Here's how the part is built. I have some questions about the finished solid (model axes, mm). A direction names the side the tool comes from. Round coordinates to 2 decimals unless told otherwise and drop trailing zeros. Loops run counter-clockwise (first coordinate to the right, second up) from the corner with the lowest first, then second, coordinate; pieces in that order, holes last. Notation, with made-up numbers: M 31.25,25.5 L 36.25,25.5 A13 cw 36.25,39.5 Z; hole C 86.5,30.25 d3. An arc over 180 degrees is marked long. Use a Markdown table: item, result.
Autodesk Inventor part; units mm, degrees
ref_plane "YZ Plane" through (0, 0, 0) normal (1, 0, 0) x (0, 1, 0)
ref_plane "XZ Plane" through (0, 0, 0) normal (0, 1, 0) x (-1, 0, 0)
ref_plane "XY Plane" through (0, 0, 0) normal (0, 0, 1) x (1, 0, 0)
sketch "Sketch1" plane through (0, 0, 0) normal (0, 0, 1) x (1, 0, 0)
  line L0 (-33, 0) -> (33, 0)
  line L1 (33, 0) -> (33, -58)
  line L2 (33, -58) -> (-33, -58)
  line L3 (-33, -58) -> (-33, 0)
  point P0 (0, 0)
  dimension "d0" = 58
  dimension "d1" = 66
  dimension "d2" = 33
  dimension "d3" = 0
extrude "clamp_base" add sketch "Sketch1" against normal blind 190
sketch "Sketch2" plane through (0, 0, 0) normal (0, 0, 1) x (1, 0, 0)
  line L0 (-25, -58) -> (25, -58)
  line L1 (25, -58) -> (25, -8)
  line L2 (25, -8) -> (-25, -8)
  line L3 (-25, -8) -> (-25, -58)
  line L4 (-33, -58) -> (33, -58)
  point P0 (0, 0)
  dimension "d6" = 50
  dimension "d7" = 50
  dimension "d8" = 25
extrude "clamp_extrusion" cut sketch "Sketch2" against normal through all
sketch "Sketch4" plane through (-33, 0, 0) normal (0, 1, 0) x (1, 0, 0)
  line L0 (-70, 190) -> (101, 190)
  line L1 (101, 190) -> (101, 0)
  line L2 (101, 0) -> (-70, 0)
  line L3 (-70, 0) -> (-70, 190)
  line L4 (66, 0) -> (0, 0)
  line L5 (0, 190) -> (66, 190)
  line L6 (0, 0) -> (0, 190)
  line L7 (66, 0) -> (66, 190)
  point P0 (33, 0)
  dimension "d35" = 0
  dimension "d36" = 0
  dimension "d37" = 70
  dimension "d38" = 35
extrude "platform" add sketch "Sketch4" along normal blind 15
sketch "Sketch8" plane through (33, -58, 0) normal (1, 0, 0) x (0, 0, -1)
  line L0 (0, 0) -> (0, 58)
  line L1 (190, 58) -> (190, 0)
  point P0 (45, 24.0271)
  point P1 (145, 24.0271)
  dimension "d51" = 45
  dimension "d60" = 100
  dimension "d61" = 190
hole "clampHole" at (33, -33.9729, -45) at (33, -33.9729, -145) direction (-1, 0, 0) diameter 10 end through all
sketch "tabWeld" plane through (-33, 15, 0) normal (0, 1, 0) x (1, 0, 0)
  line L0 (6.168, 65.1137) -> (67.4515, 116.5367)
  line L1 (-26.6142, 104.1819) -> (34.6693, 155.6049)
  line L2 (-70, 0) -> (101, 0)
  line L3 (-70, 190) -> (-70, 0)
  line L4 (6.168, 65.1137) -> (-26.6142, 104.1819)
  line L5 (-10.2231, 84.6478) -> (51.0604, 136.0708)
  line L6 (101, 0) -> (101, 190)
  line L7 (4.0276, 129.8934) -> (36.8097, 90.8252)
  line L8 (101, 190) -> (-70, 190)
  line L9 (101, 190) -> (66.0569, 219.3207)
  point P0 (33, 0)
  point P1 (20.4186, 110.3593)
  dimension "d63" = 80
  dimension "d64" = 51
  dimension "d67" = 40
  dimension "d68" = 171
  dimension "d70" = 40
  dimension "d71" = 190
  dimension "d88" = 40
  dimension "d89" = 145
ref_plane "Work Plane4" through (-28.9724, 15, -129.8934) normal (-0.766, 0, 0.6428) x (0.6428, 0, 0.766)
sketch "reelWeld" plane through (-33, 15, 0) normal (0, 1, 0) x (1, 0, 0)
  line L0 (-37.0187, 107.8529) -> (-60, 88.5693)
  line L1 (-70, 0) -> (101, 0)
  line L2 (-15.0049, 34.9462) -> (7.9765, 54.2298)
  line L3 (-70, 190) -> (-70, 0)
  line L4 (-10.2231, 84.6478) -> (51.0604, 136.0708)
  line L5 (-10.2231, 84.6478) -> (-68.0536, 36.1223)
  line L6 (-60, 88.5693) -> (-15.0049, 34.9462)
  point P0 (33, 0)
  dimension "d75" = 40
  dimension "d77" = 30
  dimension "d78" = 70
  dimension "d79" = 70
  dimension "d86" = 35
  dimension "d87" = 10
fillet "Fillet1" radius 2 2 edges at (33, 0, -95) (-33, 0, -95)
chamfer "Chamfer1" distance 2 angle 45 24 edges at (68, 15, -95) (-17.5, 15, -190) (-103, 15, -95) (-17.5, 15, 0) (51.5, 0, -190) (33, -30, -190) (68, 0, -95) (51.5, 0, 0) (33, -30, 0) (-33, -30, -190) (-69, 0, -190) (-103, 0, -95) (-69, 0, 0) (-33, -30, 0) (68, 7.5, -190) (-103, 7.5, -190) (-103, 7.5, 0) (68, 7.5, 0) (0, -8, -190) (25, -33, -190) (-25, -33, -190) (0, -8, 0) (-25, -33, 0) (25, -33, 0)
ref_plane "Work Plane5" through (-43.2231, 15, -84.6478) normal (-0.6428, 0, -0.766) x (0, -1, 0)
equation "\"d0\" = support_frame_squareBarDimension + support_baseClamp_thickness"
equation "\"d1\" = support_frame_squareBarDimension + 2 * support_baseClamp_thickness"
equation "\"d4\" = width"
equation "\"d6\" = support_frame_squareBarDimension"
equation "\"d7\" = support_frame_squareBarDimension"
equation "\"d37\" = 2 * support_baseClamp_platformLengthBuffer"
equation "\"d38\" = support_baseClamp_platformLengthBuffer"
equation "\"d13\" = support_baseClamp_platformThickness"
equation "\"d53\" = clampHoleDiameter"
equation "\"d75\" = d67"
equation "\"d79\" = d78"
equation "\"hoop_width_large\" = 51"
equation "\"width\" = clampHoleDiameter + clampHoleSpacing + 2 * buffer"
equation "\"clampHoleSpacing\" = support_frame_clampHoleSpacing"
equation "\"clampHoleDiameter\" = support_frame_clampHoleDiameter"
equation "\"d12\" = -y + r - d15"
equation "\"d15\" = hoop_width_large"
equation "\"sleeveHoleDiameter\" = support_baseClamp_sleeveHoleDiameter"
equation "\"theta\" = hoop_angle_z"
equation "\"phi\" = support_baseClamp_sleeveSweepTerminationAngle"
equation "\"support_frame_squareBarDimension\" = 50"
equation "\"support_baseClamp_thickness\" = 8"
equation "\"support_baseClamp_sleeveHoleDiameter\" = 12"
equation "\"hoop_angle_z\" = 45deg"
equation "\"support_baseClamp_sleeveSweepTerminationAngle\" = 55deg"
equation "\"support_baseClamp_platformThickness\" = 15"
equation "\"support_baseClamp_platformWidthBuffer\" = 0"
equation "\"support_baseClamp_platformLengthBuffer\" = 35"
equation "\"rack_tooth_thickness\" = 5"
equation "\"rack_tooth_addendum\" = 5"
equation "\"rack_tooth_dedendum\" = 5"
equation "\"hoop_thickness_large\" = 4"
equation "\"hoop_width_medium\" = 33.7"
equation "\"hoop_thickness_medium\" = 3.2"
equation "\"hoop_width_small\" = 25.4"
equation "\"hoop_thickness_small\" = 2"
equation "\"hoop_bearing_length\" = 5deg"
equation "\"hoop_cable_diam\" = 5"
equation "\"hoop_cable_pulley_diam\" = 22"
equation "\"secure_arm_radii\" = 9"
equation "\"secure_arm_angle\" = 35deg"
equation "\"support_frame_endHoleBuffer\" = 45"
equation "\"hoop_tabs_thickness\" = 6"
equation "\"support_frame_squareBarThickness\" = 5"
equation "\"wheelchair_deployed_length\" = 1067"
equation "\"wheelchair_deployed_height\" = 914"
equation "\"hoop_tabs_hole\" = 12"
equation "\"wheelchair_deployed_width\" = 635"
equation "\"support_frame_squareBarFillet\" = 2"
equation "\"sm_varx_pinPlate_thickness\" = 5"
equation "\"sm_varx_member_tolerance\" = 0"
equation "\"sm_varx_pinPlate_holeDiameter\" = 5"
equation "\"sm_varx_squareBarThickness\" = 2.5"
equation "\"hoop_bushing23_radialInterference\" = 0"
equation "\"hoop_bushing12_radialInterference\" = 0"
equation "\"hoop_bushing12_od\" = 43"
equation "\"wheelchatir_pos_deploy_angle_0\" = 65deg"
equation "\"wheelchatir_pos_store_angle_0\" = 90deg"
equation "\"wheelchatir_pos_deploy_angle_1\" = 20deg"
equation "\"wheelchatir_pos_store_angle_1\" = 20deg"
equation "\"hoop_bushing23_od\" = 27.3"
equation "\"hoop_bushing12_thickness\" = 9.3"
equation "\"hoop_bushing23_thickness\" = 1.9"
properties part number "support_basePart" material "Steel, High Strength, Low Alloy"
Q1. Imagine slicing it at B-B, the plane y = -46. Please give me the cut outline in (x, z), then the cut area to 3 significant figures.
Return value:
| item | result |
|---|---|
| outline | M -33,-188 L -31,-190 L -27,-190 L -25,-188 L -25,-2 L -27,0 L -31,0 L -33,-2 Z; M 25,-188 L 27,-190 L 31,-190 L 33,-188 L 33,-2 L 31,0 L 27,0 L 25,-2 Z |
| area | 3,020 mm^2 |
Q2. Imagine slicing it at A-A, the plane z = -45. Please give me the cut outline in (x, y).
Return value:
| item | result |
|---|---|
| outline | M -103,2 L -101,0 L -35,0 A2 cw -33,-2 L -33,-28.97 L -25,-28.97 L -25,-8 L 25,-8 L 25,-28.97 L 33,-28.97 L 33,-2 A2 cw 35,0 L 66,0 L 68,2 L 68,13 L 66,15 L -101,15 L -103,13 Z; M -33,-58 L -25,-58 L -25,-38.97 L -33,-38.97 Z; M 25,-58 L 33,-58 L 33,-38.97 L 25,-38.97 Z |
Q3. Imagine slicing it at D-D, the plane x = 57.5. Please give me the cut outline in (y, z), then the cut area to 3 significant figures.
Return value:
| item | result |
|---|---|
| outline | M 0,-188 L 2,-190 L 13,-190 L 15,-188 L 15,-2 L 13,0 L 2,0 L 0,-2 Z |
| area | 2,840 mm^2 |
Q4. Imagine slicing it at C-C, the plane x = -2.5. Please give me the cut outline in (y, z).
Return value:
| item | result |
|---|---|
| outline | M -8,-188 L -6,-190 L 13,-190 L 15,-188 L 15,-2 L 13,0 L -6,0 L -8,-2 Z |
Q5. Will these pins go through, and if not, where does the flat tip stop? P1, Ø11.5, axis at y = -33.97, z = -45, coming from the -X side; P2, Ø5, axis at x = -33.5, y = 0, coming from the +Z side; P3, Ø5, axis at x = -37.5, z = -68.5, coming from the -Y side; P4, Ø15, axis at x = 11, z = -69.5, coming from the -Y side.
Return value:
| item | result |
|---|---|
| P1 | stops at x = -33 |
| P2 | stops at z = 0 |
| P3 | stops at y = 0 |
| P4 | stops at y = -8 |
Q6. For faces 1 (the flat face through (0, -8, -94)), 2 (the cylindrical face through (-29, -34, -140)), 3 (the flat face through (50, 0, -96)), 4 (the flat face through (-68, 0, -96)), which set-ups out of +Z, -Z, +X, -X, +Y, -Y let a thin tool reach every point of the face, with its end or its side?
Return value:
| item | result |
|---|---|
| face 1 | +Z, -Z, -Y |
| face 2 | +X, -X |
| face 3 | +Z, -Z, +X, -Y |
| face 4 | +Z, -Z, -X, -Y |
Q7. I need wall thicknesses on line 1 (Z direction, x = -30, y = -33.5); line 2 (Y direction, x = -27, z = -45); line 3 (X direction, y = -22, z = -169.5). Which ranges of each line are inside material? Lowest first, please. Write a range as from..to.
Return value:
| item | result |
|---|---|
| line 1 | z = -190..-149.98, -140.02..-49.98, -40.02..0 |
| line 2 | y = -58..-38.97, -28.97..15 |
| line 3 | x = -33..-25, 25..33 |
Q8. We'd pull the mould along Z, two halves only. Please class faces 5 (the flat face through (-103, 7, -94)), 6 (the cylindrical face through (29, -34, -140)), 7 (the cylindrical face through (-29.056, -37.352, -41.315)), 8 (the conical face through (33.004, -0.048, -188.792)): pulls with the +Z half, pulls with the -Z half, needs draft (parallel to the pull), parting line crosses it, or undercut.
Return value:
| item | result |
|---|---|
| face 5 | needs draft |
| face 6 | undercut |
| face 7 | undercut |
| face 8 | pulls with the -Z half |
